Here's how the part is built. I have some questions about the finished solid (model axes, mm). A direction names the side the tool comes from. Give positions to 0.01 mm unless a question says otherwise; leave off trailing zeros. Loops run counter-clockwise (first coordinate to the right, second up) from the corner with the lowest first, then second, coordinate; pieces in that order, holes last. Notation, with made-up numbers: (7.25, 73) -> (36.25, 73) arc R23 ccw to (36.25, 102) -> close; hole circle Ø3 at (60.5, -15.75). An arc over 180 degrees is marked (long way). Answer in a Markdown table with one row per item. Add a question column.
Item 1: If we section it at B-B (y = -19): Write out the boundary of the cut face in (x, z).
Item 2: If we section it at A-A (z = 0): Write out the boundary of the cut face in (x, y).
Item 3: If I drill on line 1 (X direction, y = -3, z = 0); line 2 (X direction, y = -6, z = 0); line 3 (Z direction, x = 11, y = -5), over which ranges is the centre line in solid material (lowest first)?
Item 4: For P1, Ø5, axis at y = 11, z = 5.5, coming from the +X side; P2, Ø10, axis at y = -7.5, z = 23, coming from the -X side; P3, Ø1.5, axis at x = 17.5, z = -30, coming from the -Y side; P4, Ø20.5, axis at x = 39.5, z = 3.5, coming from the +Y side, each with a flat end and sliding along its axis, tell me the tip position at first contact or that it passes through.
Item 5: We'd pull the mould along X, two halves only. Please class faces 1 (the face through (-0.61, 16.76, -8.29)), 2 (the face through (26, 3.088, -28)), 3 (the face through (26, 8.288, -28)): released by +X, released by -X, zero draft, split by the parting line, or undercut.
Item 6: Which directions (+Z, -Z, +X, -X, +Y, -Y) give clear straight access to the entire face, cutting with the end or side of a thin tool? Please do faces 4 (the face through (26, 25.472, -23)), 5 (the face through (17, -5.512, 34)).
```python
from build123d import *

# Parameters (mm, degrees)
CHAMFER1_SIZE = 3.5


with BuildPart() as part:
    # Sketch1 → Revolve2 (revolve)
    with BuildSketch(Plane.XY):
        Polygon((-8.685956571, 3.088170612), (-1.885956571, 3.088170612), (-1.885956571, -22.827972222), (3.314043429, -22.827972222), (3.314043429, 25.472027778), (-1.885956571, 25.472027778), (-1.885956571, 8.288170612), (-12.185956571, 8.288170612), (-12.185956571, 3.088170612), (-12.185956571, -5.511829388), (-8.685956571, -5.511829388), align=None)
    revolve(axis=Axis((25.714043429, 25.472027778, 0), (0, -1, 0)))

    # Chamfer1
    chamfer1_edges = [part.edges().sort_by_distance(p)[0] for p in [
        (63.614043429, 8.288170612, 0),
    ]]
    chamfer(chamfer1_edges, length=CHAMFER1_SIZE)


solid = part.part
```
Recorded:
| question | item | result |
|---|---|---|
| 1 | outline | circle Ø55.2 at (25.71, 0); hole circle Ø44.8 at (25.71, 0) |
| 2 | outline | (-12.19, -5.51) -> (-8.69, -5.51) -> (-8.69, 3.09) -> (-1.89, 3.09) -> (-1.89, -22.83) -> (3.31, -22.83) -> (3.31, 25.47) -> (-1.89, 25.47) -> (-1.89, 8.29) -> (-8.69, 8.29) -> (-12.19, 4.79) -> close; (48.11, -22.83) -> (53.31, -22.83) -> (53.31, 3.09) -> (60.11, 3.09) -> (60.11, -5.51) -> (63.61, -5.51) -> (63.61, 4.79) -> (60.11, 8.29) -> (53.31, 8.29) -> (53.31, 25.47) -> (48.11, 25.47) -> close |
| 3 | line 1 | x = -12.19 to -8.69, -1.89 to 3.31, 48.11 to 53.31, 60.11 to 63.61 |
| 3 | line 2 | x = -1.89 to 3.31, 48.11 to 53.31 |
| 3 | line 3 | z = -34.93 to -31.09, -23.35 to -16.89, 16.89 to 23.35, 31.09 to 34.93 |
| 4 | P1 | stops at x = 53.15 |
| 4 | P2 | stops at x = -7.41 |
| 4 | P3 | stops at y = 3.09 |
| 4 | P4 | stops at y = 25.47 |
| 5 | face 1 | split by the parting line |
| 5 | face 2 | undercut |
| 5 | face 3 | zero draft |
| 6 | face 4 | +Z, -Z, +X, -X, +Y |
| 6 | face 5 | -Y |
